```python
from build123d import *

# Parameters (mm, degrees)
BOSS_EXTRUDE1_DEPTH = 7
SKETCH4_R           = 2.75
CUT_EXTRUDE1_DEPTH  = 40


with BuildPart() as part:
    # Sketch3 → Boss-Extrude1 (new body, symmetric)
    with BuildSketch(Plane.XY):
        Polygon((-9, 0), (-21, 0), (-21, 40), (21, 40), (21, 0), (9, 0), (9, 26.8), (-9, 26.8), align=None)
    extrude(amount=BOSS_EXTRUDE1_DEPTH, both=True)

    # Sketch4 → Cut-Extrude1 (cut)
    with BuildSketch(Plane(origin=(0, 40, 0), x_dir=(1, 0, 0), z_dir=(0, 1, 0))):
        with Locations((-16, 0)):
            Circle(SKETCH4_R)
        with Locations((16, 0)):
            Circle(SKETCH4_R)
    extrude(amount=-CUT_EXTRUDE1_DEPTH, mode=Mode.SUBTRACT)


solid = part.part
```
Model file for the job. Use its own axes, mm. A direction names the side the tool comes from. Coordinates: 2 decimals unless noted, no trailing zeros. Order: outer loops, then holes, each group sorted by start corner. A loop starts at its lowest first (then second) coordinate and runs counter-clockwise, first axis right, second up. Notation, with made-up numbers: (-31.75, 29.5) -> (19.25, 29.5) arc R23 cw to (19.25, 59.5) -> close; hole circle Ø2 at (61, 31). An arc over 180 degrees is marked (long way). Answer as a JSON object with one key per item and string values. Group by question number.
1) Which spindle directions (+Z, -Z, +X, -X, +Y, -Y) get a long thin tool onto all of the face, cutting with end or side? Do faces 5 (the face through (13.253, 20.28, -0.121)), 6 (the face through (0, 26.8, 0)). Say none if no direction does.
2) Drill centre lines: L1, parallel to X at y = 11, z = 0; L2, parallel to X at y = 20.5, z = 3.5; L3, parallel to X at y = 7, z = -2. Where is each one in solid material? Low to high.
3) Pull direction X, two halves, no side cores. Call faces 1 (the face through (-9, 14, 0)), 2 (the face through (9, 13, 0)), 3 (the face through (0, 29, 7)), 4 (the face through (21, 20, 0)): +X half, -X half, draft (parallel to the pull), parting line (faces both ways), or undercut.
4) Flat gauge pins, fed straight in: pin 1 (2 mm diameter, centred on x = 8.5, z = -3, fed in from -Y); pin 2 (4.5 mm diameter, centred on x = -16, z = 0, fed in from -Y); pin 3 (4 mm diameter, centred on x = 4, z = -3, fed in from -Y). Where does each tip first touch, or does it go through?
5) Cut at A-A, the plane y = 24.5. Write the cut outline in (x, z), then the cut area to 3 significant figures.
6) Cut at D-D, the plane y = 35. Write the cut outline in (x, z).
7) Cut at B-B, the plane z = 0. Write the cut outline in (x, y).
8) Cut at C-C, the plane x = 16. Write the cut outline in (y, z).
Check values:
{
 "1": {"face 5": "+Y, -Y", "face 6": "+Z, -Z, -Y"},
 "2": {"L1": "x = -21 to -18.75, -13.25 to -9, 9 to 13.25, 18.75 to 21", "L2": "x = -21 to -9, 9 to 21", "L3": "x = -21 to -17.89, -14.11 to -9, 9 to 14.11, 17.89 to 21"},
 "3": {"face 1": "undercut", "face 2": "undercut", "face 3": "draft", "face 4": "+X half"},
 "4": {"pin 1": "stops at y = 0", "pin 2": "passes through", "pin 3": "stops at y = 26.8"},
 "5": {"outline": "(-21, -7) -> (-9, -7) -> (-9, 7) -> (-21, 7) -> close; (9, -7) -> (21, -7) -> (21, 7) -> (9, 7) -> close; hole circle Ø5.5 at (-16, 0); hole circle Ø5.5 at (16, 0)", "area": "288 mm²"},
 "6": {"outline": "(-21, -7) -> (21, -7) -> (21, 7) -> (-21, 7) -> close; hole circle Ø5.5 at (-16, 0); hole circle Ø5.5 at (16, 0)"},
 "7": {"outline": "(-21, 0) -> (-18.75, 0) -> (-18.75, 40) -> (-21, 40) -> close; (-13.25, 0) -> (-9, 0) -> (-9, 26.8) -> (9, 26.8) -> (9, 0) -> (13.25, 0) -> (13.25, 40) -> (-13.25, 40) -> close; (18.75, 0) -> (21, 0) -> (21, 40) -> (18.75, 40) -> close"},
 "8": {"outline": "(0, -7) -> (40, -7) -> (40, -2.75) -> (0, -2.75) -> close; (0, 2.75) -> (40, 2.75) -> (40, 7) -> (0, 7) -> close"}
}
